Verification items for the finished model (mm, model axes). Face numbers are marked on the shaded views. A direction names the side the tool comes from. Give positions to 0.01 mm unless a question says otherwise; leave off trailing zeros. Write each loop counter-clockwise with the first axis right and the second up, starting at its lowest first coordinate (ties: lowest second). Pieces come first, ordered by that corner, then holes. Notation, with made-up numbers: (9, -9.5) -> (26, -9.5) arc R14 ccw to (26, -1.5) -> close; hole circle Ø6 at (-15.5, 78.25). An arc over 180 degrees is marked (long way). Answer as CSV lines item,"result".
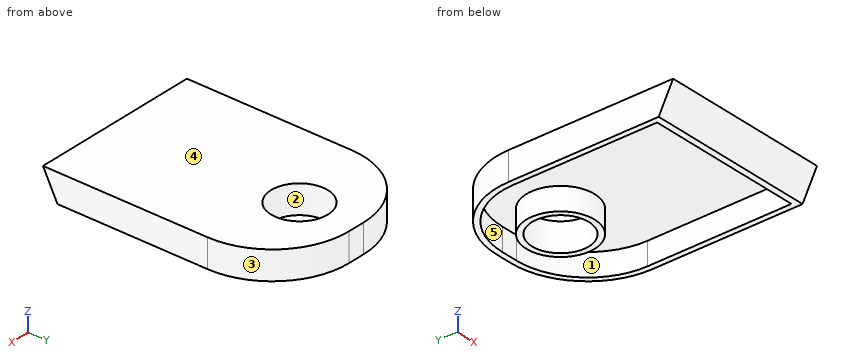
```python
from build123d import *

# Parameters (mm, degrees)
F0_W     = 38.1
F0_H     = 50.8
F0_R     = 6.35
F1_DEPTH = 6.35
F2_R     = 17.169887
F4_DEPTH = 38.1
F5_T     = -1.27


with BuildPart() as f1:
    # F0 (on Top) → F1 (new body)
    with BuildSketch(Plane.XY):
        with Locations((0, 25.4)):
            Rectangle(F0_W, F0_H)
        with Locations((0, 38.1)):
            Circle(F0_R, mode=Mode.SUBTRACT)
    extrude(amount=F1_DEPTH)

    # F2
    f2_edges = [f1.edges().sort_by_distance(p)[0] for p in [
        (-19.05, 50.8, 3.175),
        (19.05, 50.8, 3.175),
    ]]
    fillet(f2_edges, radius=F2_R)

    # F3 (on face) → F4 (join)
    with BuildSketch(Plane.YZ.offset(19.05)):
        Polygon((0, 0), (0, 6.35), (-3.235487, 6.35), align=None)
    extrude(amount=-F4_DEPTH)

    # F5
    f5_openings = [f1.faces().sort_by_distance(p)[0] for p in [
        (0, 22.821689, 0),
    ]]
    offset(amount=F5_T, openings=f5_openings)


solid = f1.part
```
1) Depth check by flat-ended pin: pin 1 (20.5 mm diameter, centred on x = 0, y = 38.1, fed in from -Z); pin 2 (1.1 mm diameter, centred on x = -0.5, z = 1.5, fed in from -Y); pin 3 (3 mm diameter, centred on x = -7.5, z = 5.5, fed in from +Y); pin 4 (10 mm diameter, centred on x = 8, y = 11, fed in from -Z). Enter the tip coordinate at first touch or a pass-through.
Reported:
pin 1,"z = 0"
pin 2,"y = -1.04"
pin 3,"y = 50.3"
pin 4,"z = 5.08"
2) Section check A-A (x = 0). Record the boundary of the cut face in (y, z).
Reported:
outline,"(-3.24, 6.35) -> (0, 0) -> (1.43, 0) -> (-1.16, 5.08) -> (30.48, 5.08) -> (30.48, 0) -> (31.75, 0) -> (31.75, 6.35) -> close; (44.45, 0) -> (45.72, 0) -> (45.72, 5.08) -> (49.53, 5.08) -> (49.53, 0) -> (50.8, 0) -> (50.8, 6.35) -> (44.45, 6.35) -> close"
3) Section check D-D (y = 10). Record the boundary of the cut face in (x, z), and give its area (3 significant figures).
Reported:
outline,"(-19.05, 0) -> (-17.78, 0) -> (-17.78, 5.08) -> (17.78, 5.08) -> (17.78, 0) -> (19.05, 0) -> (19.05, 6.35) -> (-19.05, 6.35) -> close"
area,"61.3 mm²"
4) Section check C-C (y = 38.1). Record the boundary of the cut face in (x, z), and give its area (3 significant figures).
Reported:
outline,"(-18.46, 0) -> (-17.14, 0) -> (-17.14, 5.08) -> (-7.62, 5.08) -> (-7.62, 0) -> (-6.35, 0) -> (-6.35, 6.35) -> (-18.46, 6.35) -> close; (6.35, 0) -> (7.62, 0) -> (7.62, 5.08) -> (17.14, 5.08) -> (17.14, 0) -> (18.46, 0) -> (18.46, 6.35) -> (6.35, 6.35) -> close"
area,"57.1 mm²"
5) Tool access check on the marked faces 1 and 2. Record the directions out of +Z, -Z, +X, -X, +Y, -Y that give a thin tool (end or side, any length) a straight path to the whole face; none if there is none.
Reported:
face 1,"-Z"
face 2,"+Z, -Z"
6) Scan lines: line 1 along X through (y, z) = (17, 2.5); line 2 along Y through (x, z) = (0, 4.75). Record each from-to range of solid material in increasing order.
Reported:
line 1,"-19.05 to -17.78, 17.78 to 19.05"
line 2,"-2.42 to -0.99, 30.48 to 31.75, 44.45 to 45.72, 49.53 to 50.8"
7) Section check B-B (z = 4). Record the boundary of the cut face in (x, y), and give its area (3 significant figures).
Reported:
outline,"(-19.05, -2.04) -> (19.05, -2.04) -> (19.05, 33.63) arc R17.17 ccw to (1.88, 50.8) -> (-1.88, 50.8) arc R17.17 ccw to (-19.05, 33.63) -> close; circle Ø15.24 at (0, 38.1); hole (-17.78, -0.61) -> (17.78, -0.61) -> (17.78, 33.63) arc R15.9 ccw to (1.88, 49.53) -> (-1.88, 49.53) arc R15.9 ccw to (-17.78, 33.63) -> close; hole circle Ø12.7 at (0, 38.1)"
area,"268 mm²"
8) Draft check along Y on the marked faces 3, 4 and 5. Enter one of: +Y half, -Y half, draft (parallel to the pull), parting line (faces both ways), or undercut.
Reported:
face 3,"+Y half"
face 4,"draft"
face 5,"undercut"
